from build123d import *

# Parameters (mm, degrees)
SKETCH1_R           = 14.625
BOSS_EXTRUDE1_DEPTH = 10
BOSS_EXTRUDE2_START = -0.5
SKETCH2_R           = 15.625
BOSS_EXTRUDE2_DEPTH = 0.5


with BuildPart() as part:
    # Sketch1 → Boss-Extrude1 (new body)
    with BuildSketch(Plane(origin=(0, 0, 0), x_dir=(1, 0, 0), z_dir=(0, 1, 0))):
        with Locations(Location((0, 0, 0), (0, 0, 270))):
            Circle(SKETCH1_R)
        with BuildLine():
            Line((-1.322875656, 1.5), (1.322875656, 1.5))
            ThreePointArc((1.322875656, 1.5), (0, -2), (-1.322875656, 1.5))
        make_face(mode=Mode.SUBTRACT)
    extrude(amount=BOSS_EXTRUDE1_DEPTH)

    # Sketch2 → Boss-Extrude2 (add)
    with BuildSketch(Plane(origin=(0, 10, 0), x_dir=(1, 0, 0), z_dir=(0, 1, 0)).offset(BOSS_EXTRUDE2_START)):
        with Locations(Location((0, 0, 0), (0, 0, 270))):
            Circle(SKETCH2_R)
        with BuildLine():
            Line((-1.322875656, 1.5), (1.322875656, 1.5))
            ThreePointArc((1.322875656, 1.5), (0, -2), (-1.322875656, 1.5))
        make_face(mode=Mode.SUBTRACT)
    extrude(amount=BOSS_EXTRUDE2_DEPTH)


solid = part.part
Can you work these out from the model? Positions are in its coordinate system, mm. A direction names the side the tool comes from. Coordinates: 2 decimals unless noted, no trailing zeros. Write each loop counter-clockwise with the first axis right and the second up, starting at its lowest first coordinate (ties: lowest second). Pieces come first, ordered by that corner, then holes.
Q1. Imagine slicing it at D-D, the plane x = -5.5. List the corners of the cut face in (y, z) for me (3 decimals).
Results found:
outline: (0, -13.551) - (9.5, -13.551) - (9.5, -14.625) - (10, -14.625) - (10, 14.625) - (9.5, 14.625) - (9.5, 13.551) - (0, 13.551) - close
Q2. Please list where these lines run through material, in increasing order: L1, parallel to X at y = 6.5, z = 0 (3 decimals); L2, parallel to Z at x = -12, y = 2; L3, parallel to X at y = 9.75, z = 13.5.
Results found:
L1: x = -14.625 to -2, 2 to 14.625
L2: z = -8.36 to 8.36
L3: x = -7.87 to 7.87
Q3. Imagine slicing it at B-B, the plane x = 0. List the corners of the cut face in (y, z) for me (3 decimals).
Results found:
outline: (0, -14.625) - (9.5, -14.625) - (9.5, -15.625) - (10, -15.625) - (10, -1.5) - (0, -1.5) - close; (0, 2) - (10, 2) - (10, 15.625) - (9.5, 15.625) - (9.5, 14.625) - (0, 14.625) - close
Q4. If we mould it in two halves opening along Z, with no side actions, what happens to faces 1 (the face through (4.39, 4.68, 13.95)), 2 (the face through (0, 5, 2)), 3 (the face through (0, 5, -1.5)), 4 (the face through (-3, 10, 0))? For each: +Z half, -Z half, draft (parallel to the pull), parting line (faces both ways), or undercut.
Results found:
face 1: parting line
face 2: undercut
face 3: undercut
face 4: draft
Q5. For P1, Ø0.8, axis at x = 0, y = 2.5, coming from the +Z side (3 decimals); P2, Ø3, axis at x = 9.5, y = 7, coming from the -Z side; P3, Ø2, axis at y = 6, z = -1, coming from the -X side (3 decimals), each with a flat end and sliding along its axis, tell me the tip position at first contact or that it passes through.
Results found:
P1: stops at z = 14.625
P2: stops at z = -12.24
P3: stops at x = -14.625
Q6. Imagine slicing it at C-C, the plane y = 9. List the corners of the cut face in (x, z) for me (3 decimals), plus the area to 3 significant figures.
Results found:
outline: circle Ø29.25 at (0, 0); hole (-1.323, -1.5) - (1.323, -1.5) arc R2 ccw (long way) to start
area: 660 mm2
Q7. Which directions (+Z, -Z, +X, -X, +Y, -Y) give clear straight access to the entire face, cutting with the end or side of a thin tool? Please do faces 5 (the face through (0.69, 9.75, -15.61)), 6 (the face through (-12, 9.5, 9)).
Results found:
face 5: +Y, -Y
face 6: -Y
Q8. Imagine slicing it at A-A, the plane z = 0. List the corners of the cut face in (x, y) for me (3 decimals), plus the area to 4 significant figures.
Results found:
outline: (-15.625, 9.5) - (-14.625, 9.5) - (-14.625, 0) - (-2, 0) - (-2, 10) - (-15.625, 10) - close; (2, 0) - (14.625, 0) - (14.625, 9.5) - (15.625, 9.5) - (15.625, 10) - (2, 10) - close
area: 253.5 mm2
